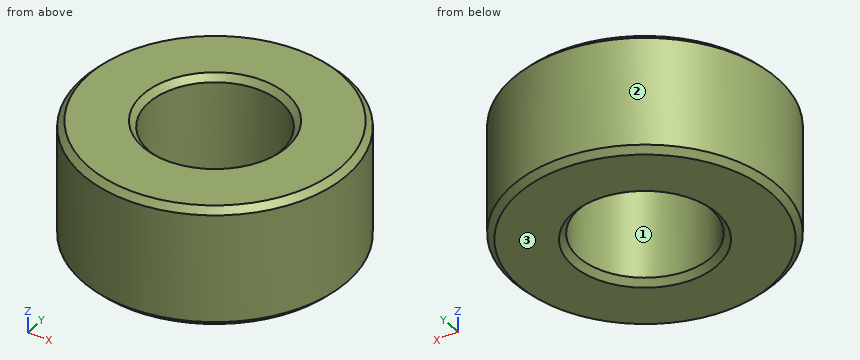
```python
from build123d import *

# Parameters (mm, degrees)
SKICA1_R                = 11
SKICA1_R_2              = 5.5
P_IDAT_VYSUNUT_M1_DEPTH = 10
ZKOSEN_1_SIZE           = 0.5


with BuildPart() as part:
    # Skica1 → Přidat vysunutím1 (new body)
    with BuildSketch(Plane.XY):
        Circle(SKICA1_R)
        Circle(SKICA1_R_2, mode=Mode.SUBTRACT)
    extrude(amount=P_IDAT_VYSUNUT_M1_DEPTH)

    # Zkosení1
    zkosen_1_edges = [part.edges().sort_by_distance(p)[0] for p in [
        (-11, 0, 0),
        (-11, 0, 10),
        (-5.5, 0, 0),
        (-5.5, 0, 10),
    ]]
    chamfer(zkosen_1_edges, length=ZKOSEN_1_SIZE)


solid = part.part
```
Geometry check sheet. Reference: the model listing, model coordinates, mm. Face numbers are marked on the shaded views. Coordinates: 2 decimals unless noted, no trailing zeros. Order: outer loops, then holes, each group sorted by start corner. A loop starts at its lowest first (then second) coordinate and runs counter-clockwise, first axis right, second up. Notation, with made-up numbers: (55, 64) - (106, 64) arc R9 ccw to (106, 74) - close; hole circle Ø3 at (43, 53.5). An arc over 180 degrees is marked (long way). Use one line per item in the form item = value.
1. Draft check along Y on the marked faces 1, 2 and 3. Enter one of: pulls with the +Y half, pulls with the -Y half, needs draft (parallel to the pull), parting line crosses it, or undercut.
Here are the results:
face_1 = undercut
face_2 = parting line crosses it
face_3 = needs draft
2. Section check A-A (x = 0). Record the boundary of the cut face in (y, z).
Here are the results:
outline = (-11, 0.5) - (-10.5, 0) - (-6, 0) - (-5.5, 0.5) - (-5.5, 9.5) - (-6, 10) - (-10.5, 10) - (-11, 9.5) - close; (5.5, 0.5) - (6, 0) - (10.5, 0) - (11, 0.5) - (11, 9.5) - (10.5, 10) - (6, 10) - (5.5, 9.5) - close
3. Gauge pin test, flat ends, axial feed: pin 1 (12 mm diameter, centred on x = -7.5, y = -1, fed in from -Z); pin 2 (3 mm diameter, centred on y = 3.5, z = 8, fed in from +X); pin 3 (5 mm diameter, centred on x = 8.5, z = 1.5, fed in from +Y). Record the tip position at first contact, or that the pin passes through.
Here are the results:
pin_1 = 0
pin_2 = 10.82
pin_3 = 9.22
4. Scan lines: line 1 (Y direction, x = 0, z = 5); line 2 (Y direction, x = 2.5, z = 2); line 3 (X direction, y = 3.5, z = 1.5). Record each from-to range of solid material in increasing order.
Here are the results:
line_1 = -11 to -5.5, 5.5 to 11
line_2 = -10.71 to -4.9, 4.9 to 10.71
line_3 = -10.43 to -4.24, 4.24 to 10.43
5. Section check C-C (z = 1.75). Record the boundary of the cut face in (x, y), then the cut area to 3 significant figures.
Here are the results:
outline = circle Ø22 at (0, 0); hole circle Ø11 at (0, 0)
area = 285 mm²
